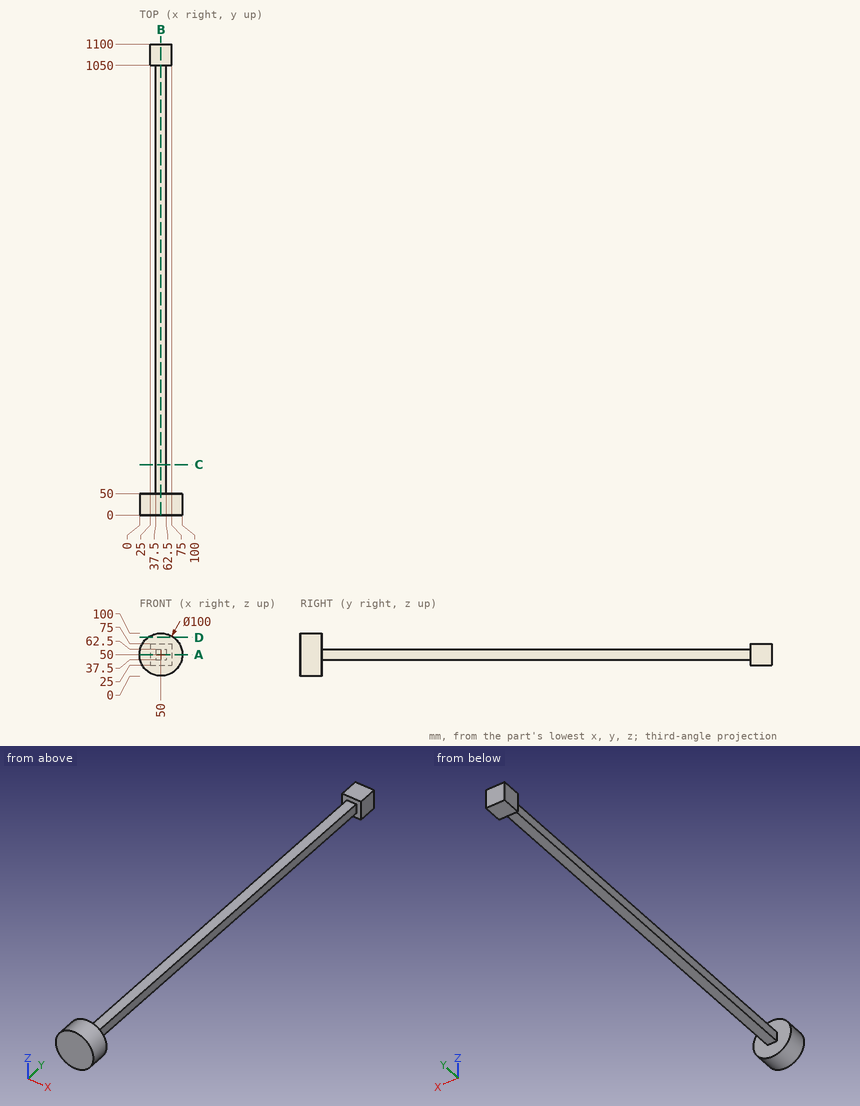
Geometry: see drawing. Coordinates: mm, zero at the bounding-box minimum. Give positions to 0.01 mm unless a question says otherwise; leave off trailing zeros. Write each loop counter-clockwise with the first axis right and the second up, starting at its lowest first coordinate (ties: lowest second). Pieces come first, ordered by that corner, then holes. Notation, with made-up numbers: M 47,28 L 99,28 A25 ccw 99,45 Z; hole C 15,24 d9. An arc over 180 degrees is marked long. Return JSON: item names as keys, results as strings. Group by question number.
1) Ray query, L1, parallel to Y at x = 34.5, z = 56.5; L2, parallel to X at y = 549, z = 40; L3, parallel to Y at x = 48, z = 85. Return the intervals inside material, ascending.
2) Cut plane A-A, the plane z = 50. Output: boundary loops of the cut face in (x, y), then the cut area to 3 significant figures.
3) First-contact query: pin 1 Ø25 at (x, y) = (52, 1085) entering from -Z; pin 2 Ø3 at (x, y) = (54.5, 758) entering from +Z; pin 3 Ø12.5 at (y, z) = (552, 54) entering from +X. Flat tips, straight axial feed; report the tip coordinate or a pass-through.
4) Cut plane B-B, the plane x = 50. Output: boundary loops of the cut face in (y, z), then the cut area to 3 significant figures.
5) Cut plane D-D, the plane z = 90. Output: boundary loops of the cut face in (x, y), then the cut area to 3 significant figures.
6) Cut plane C-C, the plane y = 118. Output: boundary loops of the cut face in (x, z).
Data:
{
 "1": {"L1": "y = 0 to 50, 1050 to 1100", "L2": "x = 37.5 to 62.5", "L3": "y = 0 to 50"},
 "2": {"outline": "M 0,0 L 100,0 L 100,50 L 62.5,50 L 62.5,1050 L 75,1050 L 75,1100 L 25,1100 L 25,1050 L 37.5,1050 L 37.5,50 L 0,50 Z", "area": "32,500 mm²"},
 "3": {"pin 1": "stops at z = 25", "pin 2": "stops at z = 62.5", "pin 3": "stops at x = 62.5"},
 "4": {"outline": "M 0,0 L 50,0 L 50,37.5 L 1050,37.5 L 1050,25 L 1100,25 L 1100,75 L 1050,75 L 1050,62.5 L 50,62.5 L 50,100 L 0,100 Z", "area": "32,500 mm²"},
 "5": {"outline": "M 20,0 L 80,0 L 80,50 L 20,50 Z", "area": "3,000 mm²"},
 "6": {"outline": "M 37.5,37.5 L 62.5,37.5 L 62.5,62.5 L 37.5,62.5 Z"}
}
